```python
from build123d import *

# Parameters (mm, degrees)
SKETCH1_W              = 82.55
SKETCH1_H              = 21.463
PLATE_DEPTH            = 1.27
SKETCH4_W              = 82.55
SKETCH4_H              = 15.24
BOSS_EXTRUDE1_DEPTH    = 1.778
SKETCH5_W              = 3.175
SKETCH5_H              = 15.24
BOSS_EXTRUDE2_DEPTH    = 19.685
BOSS_EXTRUDE5_REACH    = 84.613
SKETCH9_W              = 3.175
SKETCH9_H              = 15.24
BOSS_EXTRUDE6_REACH    = 50.618
SKETCH11_W             = 5.588
SKETCH11_H             = 15.24
CUT_EXTRUDE1_DEPTH     = 50.364623912
SKETCH13_W             = 82.55
SKETCH13_H             = 3.81
BOSS_EXTRUDE7_DEPTH    = 9.652
F_10_CLEARANCE_HOLE1_D = 5.1054
SKETCH16_W             = 6.985
SKETCH16_H             = 10.922
SKETCH16_W_2           = 9.652
CUT_EXTRUDE4_DEPTH     = 9.525
SKETCH18_W             = 1.27
SKETCH18_H             = 9.652
CUT_EXTRUDE6_DEPTH     = 52.685411423


with BuildPart() as part:
    # Sketch1 → Plate (new, symmetric)
    with BuildSketch(Plane(origin=(0, 0, 0), x_dir=(1, 0, 0), z_dir=(0, 1, 0))):
        with Locations((0, -5.1435)):
            Rectangle(SKETCH1_W, SKETCH1_H)
    extrude(amount=PLATE_DEPTH, both=True)

    # Sketch4 → Boss-Extrude1 (add)
    with BuildSketch(Plane.XY.offset(15.875)):
        with Locations((0, 8.89)):
            Rectangle(SKETCH4_W, SKETCH4_H)
    extrude(amount=-BOSS_EXTRUDE1_DEPTH)

    # Sketch5 → Boss-Extrude2 (add)
    with BuildSketch(Plane(origin=(0, 0, 14.097), x_dir=(-1, 0, 0), z_dir=(0, 0, -1))):
        with Locations((-39.6875, 8.89)):
            Rectangle(SKETCH5_W, SKETCH5_H)
        with Locations((39.6875, 8.89)):
            Rectangle(SKETCH5_W, SKETCH5_H)
    extrude(amount=BOSS_EXTRUDE2_DEPTH)

    # Sketch9 → Boss-Extrude5 (add, up to next)
    with BuildSketch(Plane.ZY.offset(-38.1), mode=Mode.PRIVATE) as boss_extrude5_sk1:
        with Locations((-4.0005, 8.89)):
            Rectangle(SKETCH9_W, SKETCH9_H)
    boss_extrude5_tool1 = extrude(boss_extrude5_sk1.sketch, amount=BOSS_EXTRUDE5_REACH, mode=Mode.PRIVATE) - part.part
    add(boss_extrude5_tool1.solids().sort_by_distance((38.1, 8.89, -4.0005))[0])

    # Sketch10 → Boss-Extrude6 (add, up to next)
    with BuildSketch(Plane(origin=(0, 0, 14.097), x_dir=(-1, 0, 0), z_dir=(0, 0, -1)), mode=Mode.PRIVATE) as boss_extrude6_sk1:
        Polygon((-8.255, 1.27), (-11.43, 1.27), (-11.43, 16.51), (-8.255, 16.51), (8.255, 16.51), (11.43, 16.51), (11.43, 1.27), (8.255, 1.27), align=None)
    boss_extrude6_tool1 = extrude(boss_extrude6_sk1.sketch, amount=BOSS_EXTRUDE6_REACH, mode=Mode.PRIVATE) - part.part
    add(boss_extrude6_tool1.solids().sort_by_distance((0, 8.89, 14.097))[0])

    # Sketch11 → Cut-Extrude1 (cut, through all)
    with BuildSketch(Plane(origin=(0, 0, -5.588), x_dir=(-1, 0, 0), z_dir=(0, 0, -1))):
        with Locations((-31.75, 8.89)):
            Rectangle(SKETCH11_W, SKETCH11_H)
        with Locations((31.75, 8.89)):
            Rectangle(SKETCH11_W, SKETCH11_H)
        with Locations((-17.78, 8.89)):
            Rectangle(SKETCH11_W, SKETCH11_H)
        with Locations((17.78, 8.89)):
            Rectangle(SKETCH11_W, SKETCH11_H)
    extrude(amount=-CUT_EXTRUDE1_DEPTH, mode=Mode.SUBTRACT)

    # Sketch13 → Boss-Extrude7 (add)
    with BuildSketch(Plane.XY.offset(15.875)):
        with Locations((0, 14.605)):
            Rectangle(SKETCH13_W, SKETCH13_H)
    extrude(amount=BOSS_EXTRUDE7_DEPTH)

    # #10 Clearance Hole1 (through all)
    with Locations(Plane(origin=(36.5125, 16.51, 20.7645), x_dir=(0, 0, 1), z_dir=(0, 1, 0))):
        with Locations((0, 0), (0.0635, -36.5125), (0.0635, -73.025)):
            Hole(F_10_CLEARANCE_HOLE1_D / 2)

    # Sketch16 → Cut-Extrude4 (cut)
    with BuildSketch(Plane(origin=(0, 0, -5.588), x_dir=(-1, 0, 0), z_dir=(0, 0, -1))):
        with Locations((-37.7825, 11.049)):
            Rectangle(SKETCH16_W, SKETCH16_H)
        with Locations((37.7825, 11.049)):
            Rectangle(SKETCH16_W, SKETCH16_H)
        with Locations((0, 11.049)):
            Rectangle(SKETCH16_W_2, SKETCH16_H)
    extrude(amount=-CUT_EXTRUDE4_DEPTH, mode=Mode.SUBTRACT)

    # Sketch18 → Cut-Extrude6 (cut, through all)
    with BuildSketch(Plane(origin=(0, 16.51, 0), x_dir=(1, 0, 0), z_dir=(0, 1, 0))):
        with Locations((-29.591, -20.701)):
            Rectangle(SKETCH18_W, SKETCH18_H)
        with Locations((-19.939, -20.701)):
            Rectangle(SKETCH18_W, SKETCH18_H)
        with Locations((19.939, -20.701)):
            Rectangle(SKETCH18_W, SKETCH18_H)
        with Locations((29.591, -20.701)):
            Rectangle(SKETCH18_W, SKETCH18_H)
    extrude(amount=-CUT_EXTRUDE6_DEPTH, mode=Mode.SUBTRACT)


solid = part.part
```
The model under review builds one solid part; all positions refer to its coordinate system, in mm. A direction names the side the tool comes from. Round coordinates to 2 decimals unless told otherwise and drop trailing zeros. Write each loop counter-clockwise with the first axis right and the second up, starting at its lowest first coordinate (ties: lowest second). Pieces come first, ordered by that corner, then holes. Notation, with made-up numbers: (24, -22) - (56, -22) arc R20 cw to (56, -9) - close; hole circle Ø3 at (-33, -23.75). An arc over 180 degrees is marked (long way). Answer as CSV lines item,"result". Start each with the question number.
(1) We need section D-D on x = 0. State the section outline as (y, z) points (3 decimals), plus the area to 3 significant figures.
(2) We need section C-C on y = 9.75. Give the number of separate pieces and of enclosed holes in the cut face, plus the area to 3 significant figures.
(3) We need section B-B on z = 9. State the section outline as (x, y) points (3 decimals).
(4) For faces 4 (the flat face through (-28.956, 13, 19)), 5 (the flat face through (25, 12.7, 21)), 6 (the flat face through (-39, 5.588, -2)), 7 (the flat face through (-13, 9, -2.413)), 8 (the flat face through (0, 11, 3.937)), list the 3-axis set-ups (+Z, -Z, +X, -X, +Y, -Y) from which the entire face can be reached by the end or side of a thin tool; tool diameter is ignored.
(5) We need section A-A on x = 16.5. State the section outline as (y, z) points (3 decimals), plus the area to 3 significant figures.
(6) To check wall thickness, follow line 1 (X direction, y = 1.5, z = -3.5) (3 decimals); line 2 (X direction, y = 12, z = 9) (3 decimals); line 3 (X direction, y = 13.75, z = 18) (3 decimals). State the ranges of each line that lie inside material, in increasing order.
(7) Draft analysis for pull direction Z (two halves, no side actions). For faces 1 (the flat face through (25, 9, -2.413)), 2 (the flat face through (19.304, 15, 21)), 3 (the flat face through (-36, 15, 25.527)), state which applies: pulls with the +Z half, pulls with the -Z half, needs draft (parallel to the pull), parting line crosses it, or undercut.
(8) For pin 1 Ø2.5 at (y, z) = (12.5, -4) entering from -X; pin 2 Ø4 at (x, y) = (32, 13.5) entering from -Z (3 decimals); pin 3 Ø1 at (x, y) = (-20, 10) entering from -Z; pin 4 Ø1.8 at (x, y) = (-36, 3.5) entering from +Z (3 decimals), all flat-tipped, find the tip position at first contact; note any pin that passes through.
Worked answers:
1,outline,"(-1.27, -5.588) - (5.588, -5.588) - (5.588, 3.937) - (16.51, 3.937) - (16.51, 18.275) - (12.7, 18.275) - (12.7, 15.875) - (-1.27, 15.875) - close; (12.7, 23.381) - (16.51, 23.381) - (16.51, 25.527) - (12.7, 25.527) - close"
1,area,"295 mm²"
2,separate pieces,"7"
2,enclosed holes,"0"
2,area,"605 mm²"
3,outline,"(-41.275, -1.27) - (41.275, -1.27) - (41.275, 16.51) - (38.1, 16.51) - (38.1, 1.27) - (11.43, 1.27) - (11.43, 16.51) - (-11.43, 16.51) - (-11.43, 1.27) - (-38.1, 1.27) - (-38.1, 16.51) - (-41.275, 16.51) - close"
4,face 4,"+Z, -Z, +Y"
4,face 5,"+Z, +X, -X, -Y"
4,face 6,"-Z, -X, +Y"
4,face 7,"+Y"
4,face 8,"-Z, +Y"
5,outline,"(-1.27, -5.588) - (1.27, -5.588) - (1.27, 15.875) - (-1.27, 15.875) - close; (12.7, 15.875) - (16.51, 15.875) - (16.51, 25.527) - (12.7, 25.527) - close"
5,area,"91.3 mm²"
6,line 1,"-41.275 to -34.544, -28.956 to -20.574, -14.986 to 14.986, 20.574 to 28.956, 34.544 to 41.275"
6,line 2,"-41.275 to -38.1, -11.43 to 11.43, 38.1 to 41.275"
6,line 3,"-41.275 to -30.226, -28.956 to -20.574, -19.304 to 19.304, 20.574 to 28.956, 30.226 to 41.275"
7,face 1,"undercut"
7,face 2,"needs draft"
7,face 3,"pulls with the +Z half"
8,pin 1,"x = -28.96"
8,pin 2,"z = 15.875"
8,pin 3,"through"
8,pin 4,"z = 15.875"
